Part print with two shaded views. Sizes in mm from the minimum x, y, z corner. Round coordinates to 2 decimals unless told otherwise and drop trailing zeros. Loops run counter-clockwise (first coordinate to the right, second up) from the corner with the lowest first, then second, coordinate; pieces in that order, holes last. Notation, with made-up numbers: (13, 49) -> (61, 49) arc R25 ccw to (61, 62) -> close; hole circle Ø4 at (-6.5, 11). An arc over 180 degrees is marked (long way). Use a Markdown table: item, result. Add a question column.
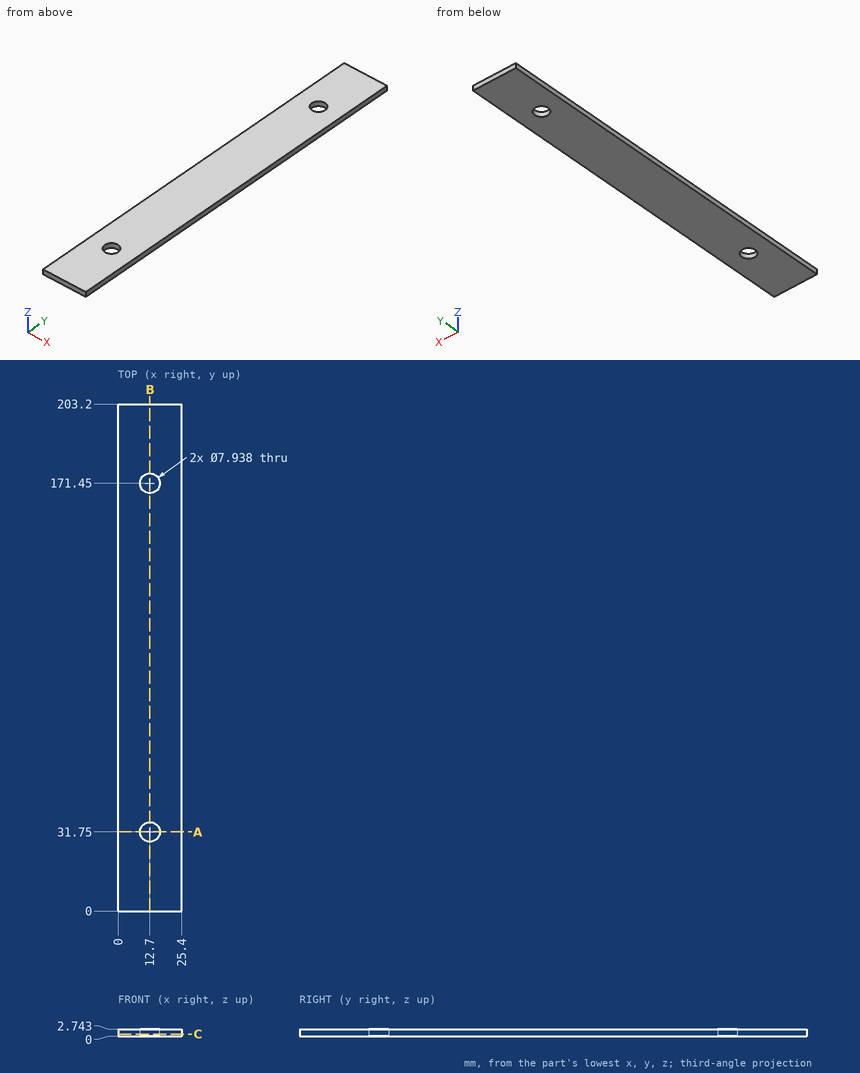
1) Wall check: probe 1 along Y at (x, z) = (12.7, 2); probe 2 along X at (y, z) = (171.45, 0.9); probe 3 along Y at (x, z) = (14, 2.35). Give the ranges that are in metal, low to high. Write a range as from..to.
2) Cut at B-B on x = 12.7. Write the cut outline in (y, z).
3) Cut at A-A on y = 31.75. Write the cut outline in (x, z).
4) Cut at C-C on z = 0.7. Write the cut outline in (x, y).
Established:
| question | item | result |
|---|---|---|
| 1 | probe 1 | y = 0..27.78, 35.72..167.48, 175.42..203.2 |
| 1 | probe 2 | x = 0..8.73, 16.67..25.4 |
| 1 | probe 3 | y = 0..28, 35.5..167.7, 175.2..203.2 |
| 2 | outline | (0, 0) -> (27.78, 0) -> (27.78, 2.74) -> (0, 2.74) -> close; (35.72, 0) -> (167.48, 0) -> (167.48, 2.74) -> (35.72, 2.74) -> close; (175.42, 0) -> (203.2, 0) -> (203.2, 2.74) -> (175.42, 2.74) -> close |
| 3 | outline | (0, 0) -> (8.73, 0) -> (8.73, 2.74) -> (0, 2.74) -> close; (16.67, 0) -> (25.4, 0) -> (25.4, 2.74) -> (16.67, 2.74) -> close |
| 4 | outline | (0, 0) -> (25.4, 0) -> (25.4, 203.2) -> (0, 203.2) -> close; hole circle Ø7.94 at (12.7, 31.75); hole circle Ø7.94 at (12.7, 171.45) |
